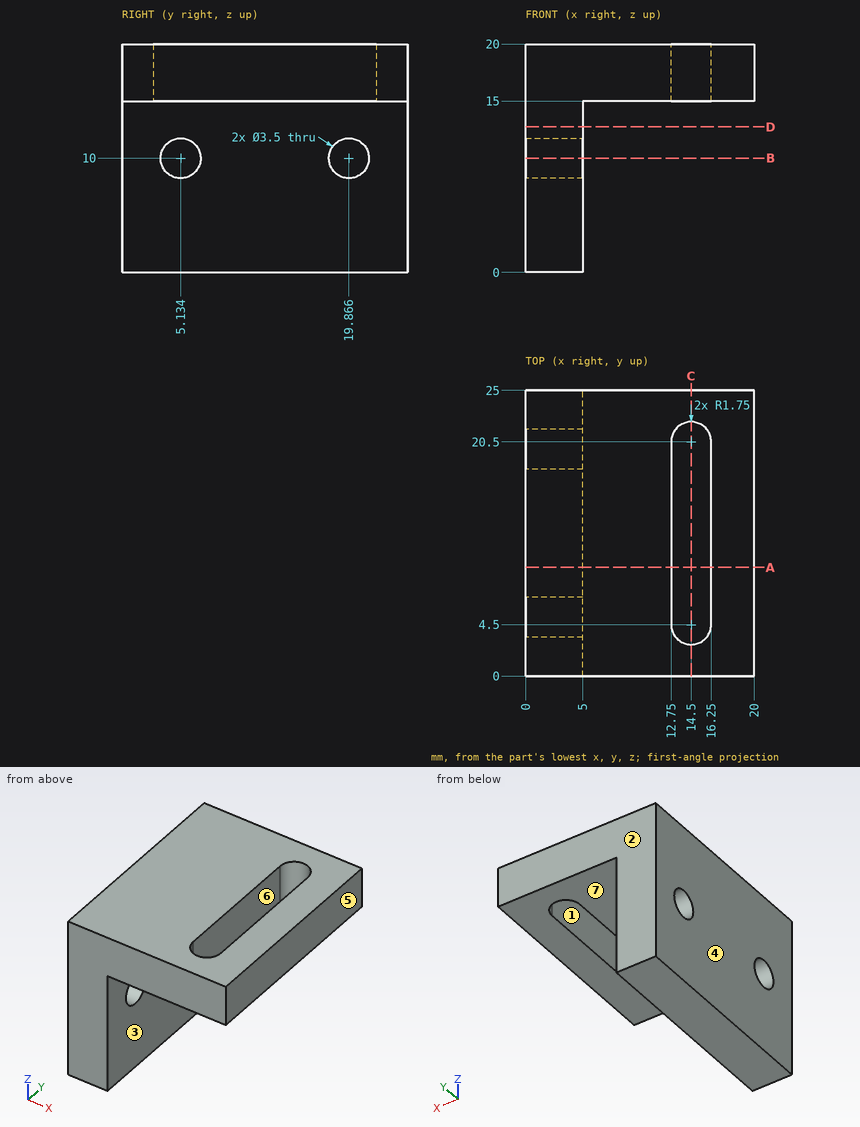
Source: three-view drawing plus pictorial views. Frame: mm from the lowest corner of the part. A direction names the side the tool comes from. Round coordinates to 2 decimals unless told otherwise and drop trailing zeros. Loops run counter-clockwise (first coordinate to the right, second up) from the corner with the lowest first, then second, coordinate; pieces in that order, holes last.
Item 1: Section B-B, the plane z = 10. Output: boundary loops of the cut face in (x, y), plus the area to 3 significant figures.
Checked values:
outline: (0, 0) - (5, 0) - (5, 3.38) - (0, 3.38) - close; (0, 6.88) - (5, 6.88) - (5, 18.12) - (0, 18.12) - close; (0, 21.62) - (5, 21.62) - (5, 25) - (0, 25) - close
area: 90.0 mm2
Item 2: Section A-A, the plane y = 9.5. Output: boundary loops of the cut face in (x, z).
Checked values:
outline: (0, 0) - (5, 0) - (5, 15) - (12.75, 15) - (12.75, 20) - (0, 20) - close; (16.25, 15) - (20, 15) - (20, 20) - (16.25, 20) - close
Item 3: Line query: L1, parallel to Y at x = 2.1, z = 10; L2, parallel to X at y = 9.75, z = 19; L3, parallel to Y at x = 2.25, z = 11. Output: solid intervals per line, ascending.
Checked values:
L1: y = 0 to 3.38, 6.88 to 18.12, 21.62 to 25
L2: x = 0 to 12.75, 16.25 to 20
L3: y = 0 to 3.7, 6.57 to 18.43, 21.3 to 25
Item 4: Section C-C, the plane x = 14.5. Output: boundary loops of the cut face in (y, z), plus the area to 3 significant figures.
Checked values:
outline: (0, 15) - (2.75, 15) - (2.75, 20) - (0, 20) - close; (22.25, 15) - (25, 15) - (25, 20) - (22.25, 20) - close
area: 27.5 mm2
Item 5: Reachability of the marked faces 5, 6 and 7 from +Z, -Z, +X, -X, +Y, -Y: full face, straight path, thin tool, end or side. Return the list, or none.
Checked values:
face 5: +Z, -Z, +X, +Y, -Y
face 6: +Z, -Z
face 7: -Z, +X, +Y, -Y
Item 6: Section D-D, the plane z = 12.75. Output: boundary loops of the cut face in (x, y), plus the area to 3 significant figures.
Checked values:
outline: (0, 0) - (5, 0) - (5, 25) - (0, 25) - close
area: 125 mm2
Item 7: Mould query, pull axis X, two halves, no side actions, for the marked faces 1, 2, 3 and 4. Classes: released by +X, released by -X, zero draft, split by the parting line, or undercut.
Checked values:
face 1: undercut
face 2: zero draft
face 3: released by +X
face 4: released by -X
Item 8: Contact query for flat-ended pins moving along their axis: P1, Ø4, axis at y = 21.5, z = 5.5, coming from the +X side; P2, Ø4.5, axis at x = 9, y = 10, coming from the -Z side. Output: stop coordinate, or through.
Checked values:
P1: stops at x = 5
P2: stops at z = 15
